Input: part model. Units: mm. Frame: model coordinates. Face numbers are marked on the shaded views. A direction names the side the tool comes from. Give positions to 0.01 mm unless a question says otherwise; leave off trailing zeros. Loops run counter-clockwise (first coordinate to the right, second up) from the corner with the lowest first, then second, coordinate; pieces in that order, holes last. Notation, with made-up numbers: (15, 73) - (45, 73) arc R12 cw to (45, 93) - close; hole circle Ø4 at (57, 1). An arc over 180 degrees is marked (long way). One line per item, written item: value.
from build123d import *

# Parameters (mm, degrees)
SKETCH1_W                 = 120.65
SKETCH1_H                 = 61.9125
BOSS_EXTRUDE1_DEPTH       = 4.7625
SKETCH2_W                 = 4.7625
SKETCH2_H                 = 12.7254
BOSS_EXTRUDE2_DEPTH       = 22.225
CUT_EXTRUDE1_REACH        = 129.448
SKETCH3_R                 = 2.25
FILLET1_R                 = 6.35
FILLET1_OF_MIRROR2_R      = 6.35
M3_CLEARANCE_SLOT1_DEPTH  = 4.7625
SKETCH7_W                 = 2.38125
SKETCH7_H                 = 10.31875
CUT_EXTRUDE3_DEPTH        = 72.353666087
CUT_EXTRUDE4_DEPTH        = 6.207125
CUT_EXTRUDE5_DEPTH        = 72.353666087
CUT_EXTRUDE6_DEPTH        = 72.353666087
M2X0_4_TAPPED_HOLE1_D     = 1.6
M2X0_4_TAPPED_HOLE1_DEPTH = 4.905375
CUT_EXTRUDE7_DEPTH        = 1.5875
M3_CLEARANCE_HOLE2_D      = 3.4
CHAMFER1_SIZE             = 0.762


# Read off the part's stored shape, not the designer's step: M3 Clearance Slot1
with BuildPart() as part:
    # Sketch1 → Boss-Extrude1 (new body)
    with BuildSketch(Plane.XY):
        Rectangle(SKETCH1_W, SKETCH1_H)
    extrude(amount=BOSS_EXTRUDE1_DEPTH)

    # Sketch2 → Boss-Extrude2 (add)
    with BuildSketch(Plane.XY.offset(4.7625)):
        with Locations((-57.94375, 2.38125)):
            Rectangle(SKETCH2_W, SKETCH2_H)
    boss_extrude2 = extrude(amount=BOSS_EXTRUDE2_DEPTH)

    # Sketch3 → Cut-Extrude1 (cut, up to next)
    with BuildSketch(Plane.ZY.offset(60.325), mode=Mode.PRIVATE) as cut_extrude1_sk1:
        with Locations((19.05, 2.36855)):
            Circle(SKETCH3_R)
    cut_extrude1_tool1 = extrude(cut_extrude1_sk1.sketch, amount=-CUT_EXTRUDE1_REACH, mode=Mode.PRIVATE) & part.part
    cut_extrude1 = cut_extrude1_tool1.solids().sort_by_distance((-60.325, 2.36855, 19.05))[0]
    add(cut_extrude1, mode=Mode.SUBTRACT)

    # Fillet1
    fillet1_edges = [part.edges().sort_by_distance(p)[0] for p in [
        (-57.94375, -3.98145, 26.9875),
        (-57.94375, 8.74395, 26.9875),
    ]]
    fillet(fillet1_edges, radius=FILLET1_R)

    # Mirror2: Boss-Extrude2, Cut-Extrude1 across plane
    add(boss_extrude2.mirror(Plane(origin=(0, 0, 0), x_dir=(0, 0, 1), z_dir=(1, 0, 0))))
    add(cut_extrude1.mirror(Plane(origin=(0, 0, 0), x_dir=(0, 0, 1), z_dir=(1, 0, 0))), mode=Mode.SUBTRACT)

    # Fillet1 of Mirror2
    fillet1_of_mirror2_edges = [part.edges().sort_by_distance(p)[0] for p in [
        (57.94375, -3.98145, 26.9875),
        (57.94375, 8.74395, 26.9875),
    ]]
    fillet(fillet1_of_mirror2_edges, radius=FILLET1_OF_MIRROR2_R)

    # M3 Clearance Slot1 outline → M3 Clearance Slot1 (cut)
    with BuildSketch(Plane.XY):
        with BuildLine():
            ThreePointArc((0.386099968, 1.50675), (2.086099968, 3.20675), (0.386099968, 4.90675))
            Line((0.386099968, 4.90675), (-0.386099968, 4.90675))
            ThreePointArc((-0.386099968, 4.90675), (-2.086099968, 3.20675), (-0.386099968, 1.50675))
            Line((-0.386099968, 1.50675), (0.386099968, 1.50675))
        make_face()
        with BuildLine():
            ThreePointArc((0.386099968, 20.55675), (2.086099968, 22.25675), (0.386099968, 23.95675))
            Line((0.386099968, 23.95675), (-0.386099968, 23.95675))
            ThreePointArc((-0.386099968, 23.95675), (-2.086099968, 22.25675), (-0.386099968, 20.55675))
            Line((-0.386099968, 20.55675), (0.386099968, 20.55675))
        make_face()
    extrude(amount=M3_CLEARANCE_SLOT1_DEPTH, mode=Mode.SUBTRACT)

    # Sketch7 → Cut-Extrude3 (cut, through all)
    with BuildSketch(Plane.XY.offset(4.7625)):
        with Locations((-59.134375, 13.903325)):
            Rectangle(SKETCH7_W, SKETCH7_H)
        with Locations((-59.134375, -9.140825)):
            Rectangle(SKETCH7_W, SKETCH7_H)
    cut_extrude3 = extrude(amount=-CUT_EXTRUDE3_DEPTH, mode=Mode.SUBTRACT)

    # Sketch8 → Cut-Extrude4 (cut)
    with BuildSketch(Plane.ZY.offset(60.325)):
        with BuildLine():
            Line((0, 8.74395), (0, -3.98145))
            Line((0, -3.98145), (20.6375, -3.98145))
            ThreePointArc((20.6375, -3.98145), (25.127628061, -2.121578061), (26.9875, 2.36855))
            Line((26.9875, 2.36855), (26.9875, 2.39395))
            ThreePointArc((26.9875, 2.39395), (25.127628061, 6.884078061), (20.6375, 8.74395))
            Line((20.6375, 8.74395), (0, 8.74395))
        make_face()
    cut_extrude4 = extrude(amount=-CUT_EXTRUDE4_DEPTH, mode=Mode.SUBTRACT)

    # Sketch11 → Cut-Extrude5 (cut, through all)
    with BuildSketch(Plane.XY.offset(4.7625)):
        with BuildLine():
            Line((-19.217596834, 2.839806331), (-44.617596834, 15.539806331))
            ThreePointArc((-44.617596834, 15.539806331), (-47.706696281, 15.400816317), (-49.2125, 12.7))
            Line((-49.2125, 12.7), (-49.2125, -12.7))
            ThreePointArc((-49.2125, -12.7), (-47.706696281, -15.400816317), (-44.617596834, -15.539806331))
            Line((-44.617596834, -15.539806331), (-19.217596834, -2.839806331))
            ThreePointArc((-19.217596834, -2.839806331), (-17.4625, 0), (-19.217596834, 2.839806331))
        make_face()
    cut_extrude5 = extrude(amount=-CUT_EXTRUDE5_DEPTH, mode=Mode.SUBTRACT)

    # Sketch12 → Cut-Extrude6 (cut, through all)
    with BuildSketch(Plane.XY.offset(4.7625)):
        with BuildLine():
            Line((-47.457403166, 20.972693669), (-22.057403166, 8.272693669))
            ThreePointArc((-22.057403166, 8.272693669), (-18.968303719, 8.411683683), (-17.4625, 11.1125))
            Line((-17.4625, 11.1125), (-17.4625, 23.8125))
            ThreePointArc((-17.4625, 23.8125), (-18.39243597, 26.05756403), (-20.6375, 26.9875))
            Line((-20.6375, 26.9875), (-46.0375, 26.9875))
            ThreePointArc((-46.0375, 26.9875), (-49.127565542, 24.541965523), (-47.457403166, 20.972693669))
        make_face()
        with BuildLine():
            Line((-20.6375, -26.9875), (-46.0375, -26.9875))
            ThreePointArc((-46.0375, -26.9875), (-49.127565542, -24.541965523), (-47.457403166, -20.972693669))
            Line((-47.457403166, -20.972693669), (-22.057403166, -8.272693669))
            ThreePointArc((-22.057403166, -8.272693669), (-18.968303719, -8.411683683), (-17.4625, -11.1125))
            Line((-17.4625, -11.1125), (-17.4625, -23.8125))
            ThreePointArc((-17.4625, -23.8125), (-18.39243597, -26.05756403), (-20.6375, -26.9875))
        make_face()
    cut_extrude6 = extrude(amount=-CUT_EXTRUDE6_DEPTH, mode=Mode.SUBTRACT)

    # M2x0.4 Tapped Hole1
    with Locations(Plane.ZY.offset(54.117875)):
        with Locations((2.38125, 7.14375), (2.38125, -0.79375)):
            m2x0_4_tapped_hole1 = Hole(M2X0_4_TAPPED_HOLE1_D / 2, depth=M2X0_4_TAPPED_HOLE1_DEPTH)

    # Mirror4: Cut-Extrude5, Cut-Extrude6 across plane
    add(cut_extrude5.mirror(Plane(origin=(0, 0, 0), x_dir=(0, 0, 1), z_dir=(1, 0, 0))), mode=Mode.SUBTRACT)
    add(cut_extrude6.mirror(Plane(origin=(0, 0, 0), x_dir=(0, 0, 1), z_dir=(1, 0, 0))), mode=Mode.SUBTRACT)

    # Mirror3: Cut-Extrude3, Cut-Extrude4, M2x0.4 Tapped Hole1 across plane
    add(cut_extrude3.mirror(Plane(origin=(0, 0, 0), x_dir=(0, 0, 1), z_dir=(1, 0, 0))), mode=Mode.SUBTRACT)
    add(cut_extrude4.mirror(Plane(origin=(0, 0, 0), x_dir=(0, 0, 1), z_dir=(1, 0, 0))), mode=Mode.SUBTRACT)
    add(m2x0_4_tapped_hole1.mirror(Plane(origin=(0, 0, 0), x_dir=(0, 0, 1), z_dir=(1, 0, 0))), mode=Mode.SUBTRACT)

    # Sketch13 → Cut-Extrude7 (cut)
    with BuildSketch(Plane.XY.offset(4.7625)):
        with BuildLine():
            Line((-16.7386, 30.95625), (-16.7386, -1.55575))
            ThreePointArc((-16.7386, -1.55575), (-15.94485, -2.3495), (-15.1511, -1.55575))
            Line((-15.1511, -1.55575), (15.1511, -1.55575))
            ThreePointArc((15.1511, -1.55575), (15.94485, -2.3495), (16.7386, -1.55575))
            Line((16.7386, -1.55575), (16.7386, 30.95625))
            Line((16.7386, 30.95625), (-16.7386, 30.95625))
        make_face()
    extrude(amount=-CUT_EXTRUDE7_DEPTH, mode=Mode.SUBTRACT)

    # M3 Clearance Hole2 (through all)
    with Locations(Plane.XY.offset(4.7625)):
        with Locations((-55.5625, 25.4), (-55.5625, -25.4), (0, -25.4), (55.5625, 25.4), (55.5625, -25.4)):
            Hole(M3_CLEARANCE_HOLE2_D / 2)

    # Chamfer1
    chamfer1_edges = [part.edges().sort_by_distance(p)[0] for p in [
        (0, 30.95625, 0),
    ]]
    chamfer(chamfer1_edges, length=CHAMFER1_SIZE)


solid = part.part
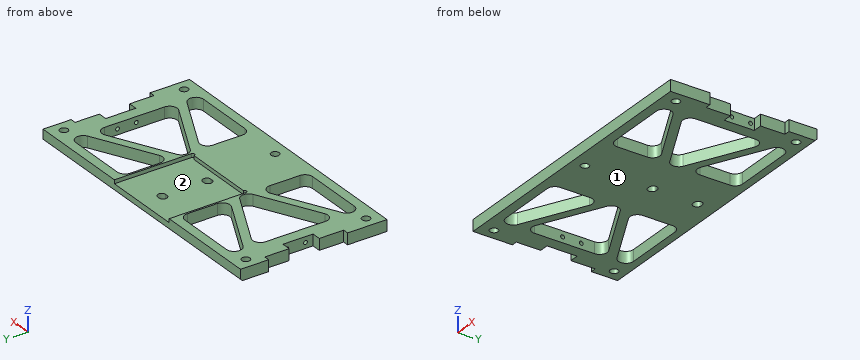
Item 1: Section C-C, the plane x = -27. Output: boundary loops of the cut face in (y, z).
Verdict:
outline: (-30.96, 0) - (-26.99, 0) - (-26.99, 4.76) - (-30.96, 4.76) - close; (-10.74, 0) - (-6.73, 0) - (-6.73, 4.76) - (-10.74, 4.76) - close; (6.73, 0) - (10.74, 0) - (10.74, 4.76) - (6.73, 4.76) - close; (26.99, 0) - (30.19, 0) - (30.96, 0.76) - (30.96, 4.76) - (26.99, 4.76) - close
Item 2: Pin query (flat end, axial travel): P1, Ø2, axis at y = 18, z = 3, coming from the +X side; P2, Ø1.8, axis at y = -0.79, z = 2.38, coming from the +X side; P3, Ø0.5, axis at x = -1, z = 3.5, coming from the +Y side. Return the tip coordinate at first contact, or that it passes through.
Verdict:
P1: stops at x = 57.94
P2: stops at x = 54.12
P3: stops at y = -1.56
Item 3: Access query for the marked faces 1 and 2. Directions: +Z, -Z, +X, -X, +Y, -Y. A direction counts if a zero-diameter tool reaches every point of the face in a straight line with its end or side. Return the directions, or none.
Verdict:
face 1: -Z, +X, -X, +Y, -Y
face 2: +Z, +Y
Item 4: Section D-D, the plane y = -25.4. Output: boundary loops of the cut face in (x, z) (1 decimal).
Verdict:
outline: (-60.3, 0) - (-57.3, 0) - (-57.3, 4.8) - (-60.3, 4.8) - close; (-53.9, 0) - (-48.8, 0) - (-48.8, 4.8) - (-53.9, 4.8) - close; (-17.9, 0) - (-1.7, 0) - (-1.7, 4.8) - (-17.9, 4.8) - close; (1.7, 0) - (17.9, 0) - (17.9, 4.8) - (1.7, 4.8) - close; (48.8, 0) - (53.9, 0) - (53.9, 4.8) - (48.8, 4.8) - close; (57.3, 0) - (60.3, 0) - (60.3, 4.8) - (57.3, 4.8) - close
Item 5: Section A-A, the plane x = -4.5. Output: boundary loops of the cut face in (y, z) (1 decimal), and give its area (3 significant figures).
Verdict:
outline: (-31, 0) - (30.2, 0) - (31, 0.8) - (31, 3.2) - (-1.6, 3.2) - (-1.6, 4.8) - (-31, 4.8) - close
area: 243 mm^2
Item 6: Material intervals for L1, parallel to Y at x = 0, z = 1.25; L2, parallel to Y at x = 54.5, z = 2.6; L3, parallel to X at y = 1.5, z = 3.4, sorted ascending.
Verdict:
L1: y = -30.96 to -27.1, -23.7 to 1.51, 4.91 to 20.56, 23.96 to 30.96
L2: y = -30.96 to -26.73, -24.07 to -3.98, 8.74 to 24.07, 26.73 to 30.96
L3: x = -54.12 to -49.21, -17.84 to -16.74, 16.74 to 17.84, 49.21 to 54.12
Item 7: Section B-B, the plane y = 25.4. Output: boundary loops of the cut face in (x, z) (1 decimal), and give its area (3 significant figures).
Verdict:
outline: (-60.3, 0) - (-57.3, 0) - (-57.3, 4.8) - (-60.3, 4.8) - close; (-53.9, 0) - (-48.8, 0) - (-48.8, 4.8) - (-53.9, 4.8) - close; (-17.9, 0) - (17.9, 0) - (17.9, 4.8) - (16.7, 4.8) - (16.7, 3.2) - (-16.7, 3.2) - (-16.7, 4.8) - (-17.9, 4.8) - close; (48.8, 0) - (53.9, 0) - (53.9, 4.8) - (48.8, 4.8) - close; (57.3, 0) - (60.3, 0) - (60.3, 4.8) - (57.3, 4.8) - close
area: 195 mm^2
